The figure shows three views and two pictorial views of one solid part (mm, origin at its lowest corner). Answer the questions. A direction names the side the tool comes from. Coordinates: 2 decimals unless noted, no trailing zeros. Write each loop counter-clockwise with the first axis right and the second up, starting at its lowest first coordinate (ties: lowest second). Pieces come first, ordered by that corner, then holes.
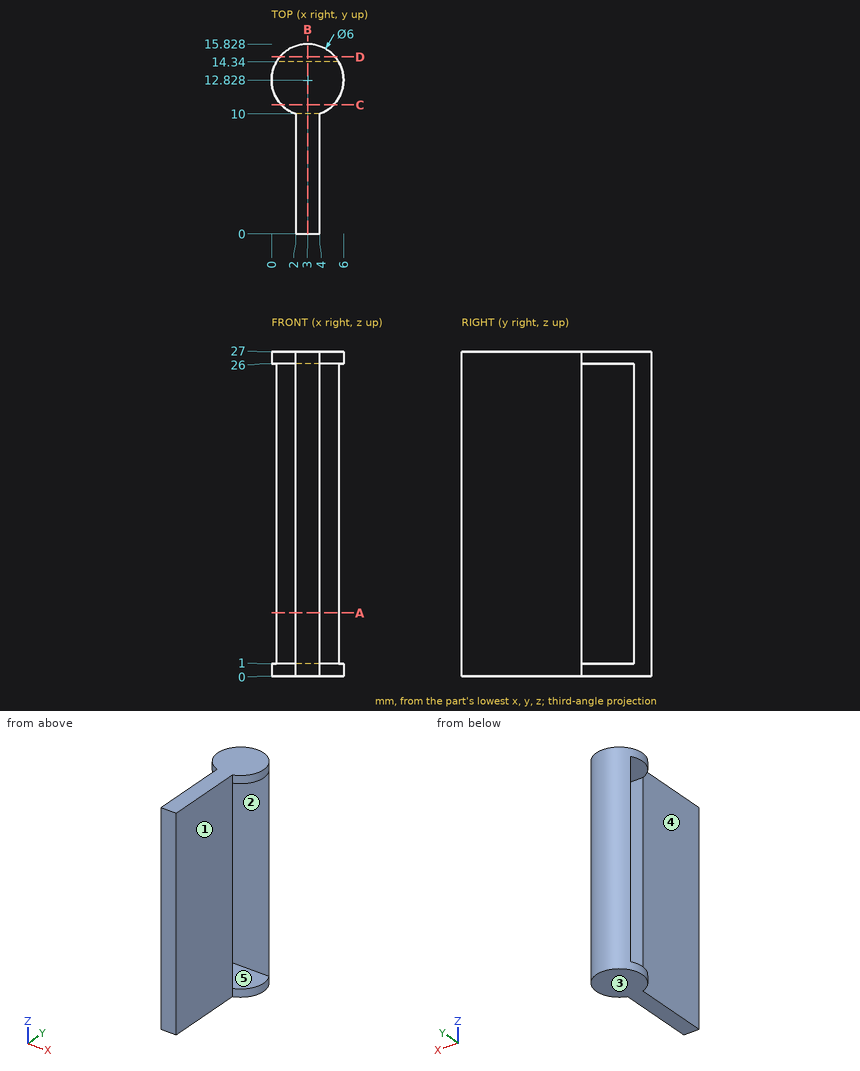
Q1. Determine the mould class of the marked faces 4 and 5 for opening direction Y: released by +Y, released by -Y, zero draft, split by the parting line, or undercut.
Answers below:
face 4: zero draft
face 5: undercut
Q2. The part is cut by section D-D, the plane y = 14.75. Write down the section's boundary in (x, z), then the cut area to 3 significant figures.
Answers below:
outline: (0.7, 0) - (5.3, 0) - (5.3, 27) - (0.7, 27) - close
area: 124 mm2
Q3. Find the intervals of material crossed by probe 1 along Z at (x, y) = (5.1, 12); probe 2 along Y at (x, z) = (2.8, 8.75); probe 3 along X at (y, z) = (9, 19.5), in increasing order.
Answers below:
probe 1: z = 0 to 1, 26 to 27
probe 2: y = 0 to 10, 14.34 to 15.82
probe 3: x = 2 to 4
Q4. Which of the six approach directions +Z, -Z, +X, -X, +Y, -Y give full straight-line access (tool end or side, diameter ignored) to the marked faces 1, 2 and 3?
Answers below:
face 1: +Z, -Z, +X, -Y
face 2: +X, -X
face 3: -Z, +X, -X, +Y, -Y
Q5. The part is cut by section A-A, the plane z = 5.25. Write down the section's boundary in (x, y).
Answers below:
outline: (0.41, 14.34) - (5.59, 14.34) arc R3 ccw to start; (2, 0) - (4, 0) - (4, 10) - (2, 10) - close
Q6. The part is cut by section C-C, the plane y = 10.75. Write down the section's boundary in (x, z).
Answers below:
outline: (0.84, 0) - (5.16, 0) - (5.16, 1) - (0.84, 1) - close; (0.84, 26) - (5.16, 26) - (5.16, 27) - (0.84, 27) - close
Q7. Given pin 1 (5 mm diameter, centred on y = 3.5, z = 18, fed in from -X); pin 2 (3 mm diameter, centred on y = 2, z = 13.5, fed in from +X), each flat-ended and moving along its own axis, determine where each tip first touches the part or whether it passes through.
Answers below:
pin 1: stops at x = 2
pin 2: stops at x = 4
Q8. The part is cut by section B-B, the plane x = 3. Write down the section's boundary in (y, z), then the cut area to 3 significant figures.
Answers below:
outline: (0, 0) - (15.83, 0) - (15.83, 27) - (0, 27) - close; hole (10, 1) - (14.34, 1) - (14.34, 26) - (10, 26) - close
area: 319 mm2
